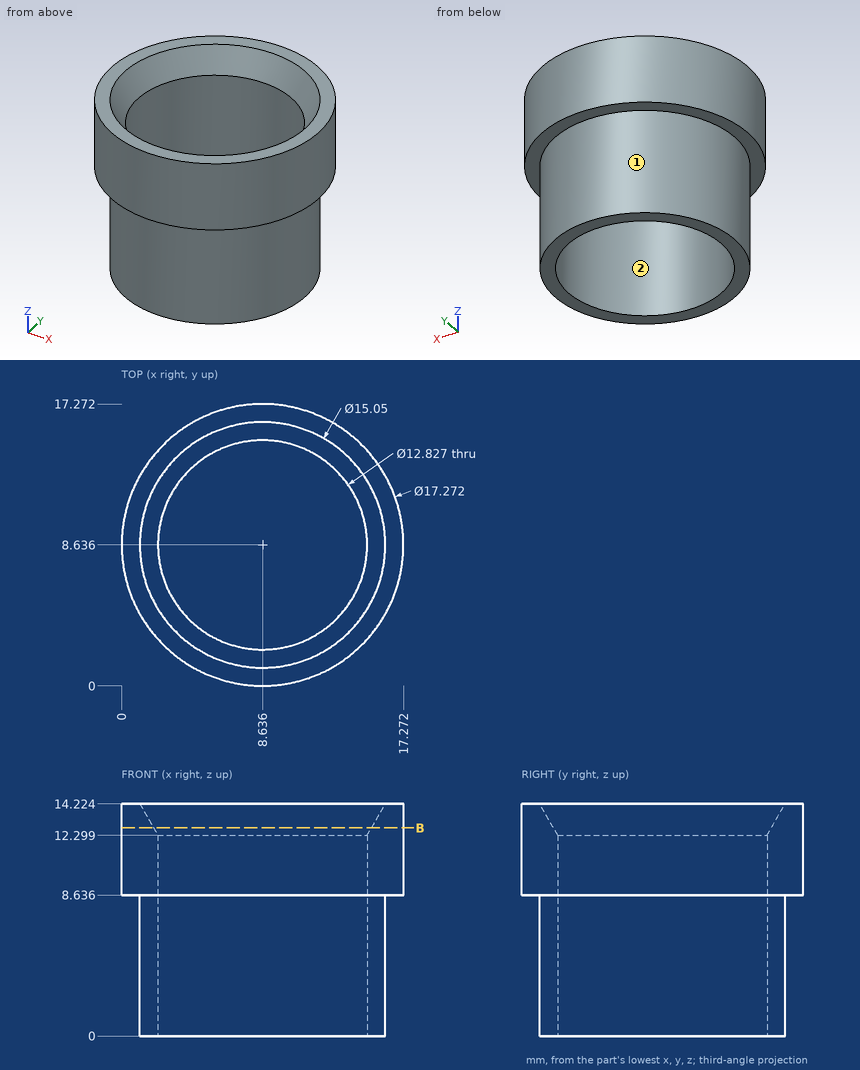
Geometry: see drawing. Coordinates: mm, zero at the bounding-box minimum. Coordinates: 2 decimals unless noted, no trailing zeros. Loops run counter-clockwise (first coordinate to the right, second up) from the corner with the lowest first, then second, coordinate; pieces in that order, holes last. Notation, with made-up numbers: (15, -20.75) -> (37, -20.75) arc R34 cw to (37, 14.25) -> close; hole circle Ø9 at (65, -32). An arc over 180 degrees is marked (long way). Write item = value, one per line. Start each with the question number.
Item 1: Mould query, pull axis X, two halves, no side actions, for the marked faces 1 and 2. Classes: pulls with the +X half, pulls with the -X half, needs draft (parallel to the pull), parting line crosses it, or undercut.
Item 2: Cut plane B-B, the plane z = 12.75. Return loops of the section in (x, y) (1 decimal).
Item 3: First-contact query: P1, Ø3, axis at y = 11.5, z = 1.5, coming from the -X side; P2, Ø5, axis at y = 13.5, z = 12.5, coming from the -X side; P3, Ø1, axis at x = 4.5, y = 10.5, coming from the -Z side; P4, Ø1, axis at x = 9.5, z = 8.5, coming from the -Y side. Flat tips, straight axial feed; report the tip coordinate or a pass-through.
Item 4: Material intervals for line 1 (X direction, y = 13.75, z = 9) (1 decimal); line 2 (Z direction, x = 15, y = 13.25) (1 decimal); line 3 (X direction, y = 3.75, z = 1) (1 decimal), sorted ascending.
Ans:
q1.face_1 = parting line crosses it
q1.face_2 = undercut
q2.outline = circle Ø17.3 at (8.6, 8.6); hole circle Ø13.3 at (8.6, 8.6)
q3.P1 = 1.24
q3.P2 = 0.33
q3.P3 = through
q3.P4 = 0.01
q4.line_1 = 1.7 to 4.8, 12.5 to 15.6
q4.line_2 = 8.6 to 14.2
q4.line_3 = 2.9 to 4.5, 12.8 to 14.4
